Answer from the drawing. Dimensions are ordinates in mm from the lowest x, y and z of the part. A direction names the side the tool comes from. Give positions to 0.01 mm unless a question says otherwise; leave off trailing zeros. Loops run counter-clockwise (first coordinate to the right, second up) from the corner with the lowest first, then second, coordinate; pieces in that order, holes last.
Item 1: Section C-C, the plane z = 31 is taken. Give the vertices of the cut face in (x, y), and give its area (3 significant figures).
Item 2: Each of these flat-tipped pins is pushed along its axis until it touches: pin 1 Ø12 at (y, z) = (25.5, 163.5) entering from -X; pin 2 Ø5 at (x, z) = (68, 148) entering from -Y; pin 3 Ø1.5 at (y, z) = (107.5, 79) entering from -X; pin 4 Ø2 at (x, y) = (90, 103.5) entering from +Z. Where does it stop, or does it pass through?
Item 3: Section A-A, the plane y = 79.5 is taken. Give the vertices of the cut face in (x, z).
Item 4: A tool of negligible diameter and unlimited length cuts with its end or side. For the marked faces 1, 2, 3, 4 and 5, from which of +Z, -Z, +X, -X, +Y, -Y can it reach the whole face along a straight path? Write none if from no direction.
Item 5: Consider line 1 along X through (y, z) = (32, 34.5); line 2 along Y through (x, z) = (66.5, 171.5). Determine where each line is inside the solid, lowest interval first.
Item 6: Section B-B, the plane x = 77 is taken. Give the vertices of the cut face in (y, z).
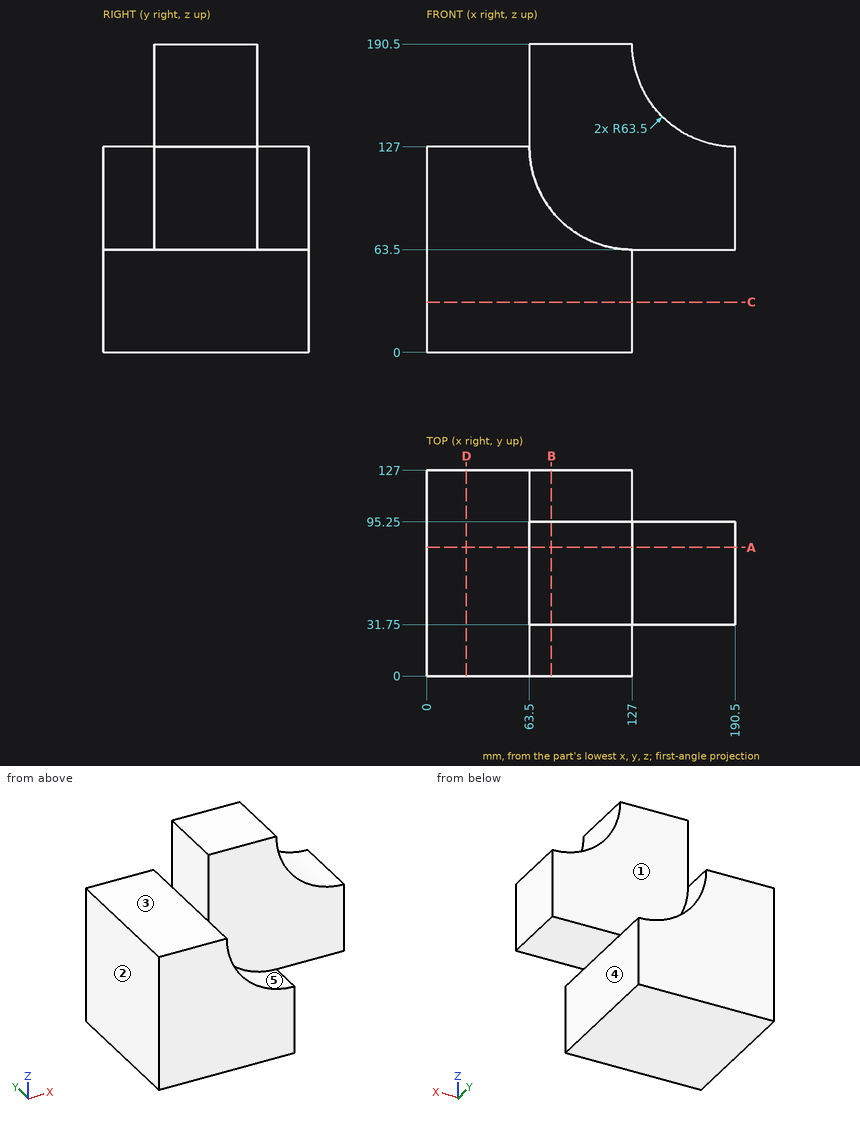
Worked answers:
1. outline: (0, 0) - (127, 0) - (127, 127) - (0, 127) - close
1. area: 16,100 mm2
2. pin 1: passes through
2. pin 2: stops at y = 31.75
2. pin 3: stops at x = 0
2. pin 4: stops at z = 76.13
3. outline: (0, 0) - (127, 0) - (127, 63.5) - (190.5, 63.5) - (190.5, 127) arc R63.5 cw to (127, 190.5) - (63.5, 190.5) - (63.5, 127) - (0, 127) - close
4. face 1: +Z, +X, +Y
4. face 2: +Z, -Z, -X, +Y, -Y
4. face 3: +Z, -X, +Y, -Y
4. face 4: -Z, +X, +Y, -Y
4. face 5: +Z, +X, -Y
5. line 1: x = 0 to 127
5. line 2: y = 31.75 to 95.25
6. outline: (0, 0) - (127, 0) - (127, 87.86) - (95.25, 87.86) - (95.25, 190.5) - (31.75, 190.5) - (31.75, 87.86) - (0, 87.86) - close
